```python
from build123d import *

# Parameters (mm, degrees)
F0_W     = 30
F0_H     = 16
F1_DEPTH = 16
F2_W     = 7
F2_H     = 6
F3_DEPTH = 6
F4_R     = 2.5
F5_DEPTH = 5


with BuildPart() as f1:
    # F0 (on Top) → F1 (new body)
    with BuildSketch(Plane.XY):
        with Locations((15, -8)):
            Rectangle(F0_W, F0_H)
    extrude(amount=F1_DEPTH)

    # F2 (on face) → F3 (join)
    with BuildSketch(Plane.XY.offset(16)):
        with Locations((15, -8)):
            Rectangle(F2_W, F2_H)
    extrude(amount=F3_DEPTH)

    # F4 (on face) → F5 (join)
    with BuildSketch(Plane.XZ.offset(16)):
        with Locations((15, 8)):
            Circle(F4_R)
    extrude(amount=F5_DEPTH)


solid = f1.part
```
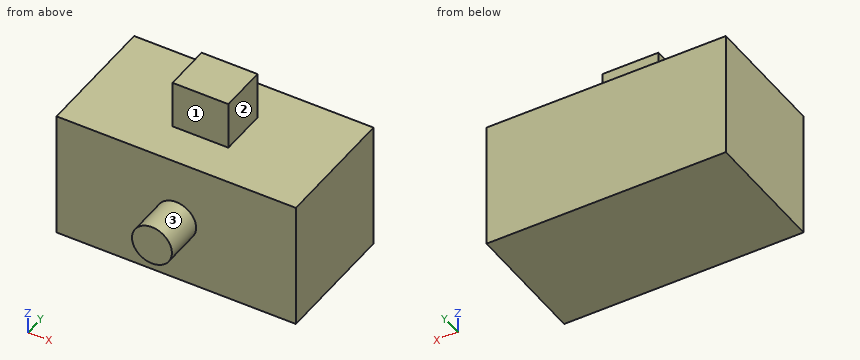
Geometry: final body of the model. Coordinates: model frame, mm. Face numbers are marked on the shaded views. A direction names the side the tool comes from. Coordinates: 2 decimals unless noted, no trailing zeros. Order: outer loops, then holes, each group sorted by start corner. A loop starts at its lowest first (then second) coordinate and runs counter-clockwise, first axis right, second up. Notation, with made-up numbers: (66, 53) -> (118, 53) arc R12 cw to (118, 57) -> close; hole circle Ø1 at (49, 79). An arc over 180 degrees is marked (long way). Use CSV: the item, a comma, the result in double quotes.
1) Section D-D on z = 3.25. Output: boundary loops of the cut face in (x, y).
Findings:
outline,"(0, -16) -> (30, -16) -> (30, 0) -> (0, 0) -> close"
2) Pin query (flat end, axial travel): pin 1 Ø8 at (x, z) = (22.5, 7) entering from -Y; pin 2 Ø3 at (y, z) = (-9.5, 18.5) entering from +X; pin 3 Ø3 at (x, z) = (16.5, 19.5) entering from +Y. Return the tip coordinate at first contact, or that it passes through.
Findings:
pin 1,"stops at y = -16"
pin 2,"stops at x = 18.5"
pin 3,"stops at y = -5"
3) Section A-A on x = 15. Output: boundary loops of the cut face in (y, z).
Findings:
outline,"(-21, 5.5) -> (-16, 5.5) -> (-16, 0) -> (0, 0) -> (0, 16) -> (-5, 16) -> (-5, 22) -> (-11, 22) -> (-11, 16) -> (-16, 16) -> (-16, 10.5) -> (-21, 10.5) -> close"
4) Line query: line 1 (Z direction, x = 26.75, y = -4.25); line 2 (Y direction, x = 1.75, z = 9.75); line 3 (X direction, y = -10, z = 19.75). Output: solid intervals per line, ascending.
Findings:
line 1,"z = 0 to 16"
line 2,"y = -16 to 0"
line 3,"x = 11.5 to 18.5"
5) Access query for the marked faces 1, 2 and 3. Directions: +Z, -Z, +X, -X, +Y, -Y. A direction counts if a zero-diameter tool reaches every point of the face in a straight line with its end or side. Return the directions, or none.
Findings:
face 1,"+Z, +X, -X, -Y"
face 2,"+Z, +X, +Y, -Y"
face 3,"-Y"
6) Section C-C on y = -18. Output: boundary loops of the cut face in (x, z), then the cut area to 3 significant figures.
Findings:
outline,"circle Ø5 at (15, 8)"
area,"19.6 mm^2"
7) Section B-B on z = 8. Output: boundary loops of the cut face in (x, y), then the cut area to 3 significant figures.
Findings:
outline,"(0, -16) -> (12.5, -16) -> (12.5, -21) -> (17.5, -21) -> (17.5, -16) -> (30, -16) -> (30, 0) -> (0, 0) -> close"
area,"505 mm^2"
